The model under review builds one solid part; all positions refer to its coordinate system, in mm. Give positions to 0.01 mm unless a question says otherwise; leave off trailing zeros. Write each loop counter-clockwise with the first axis right and the second up, starting at its lowest first coordinate (ties: lowest second). Pieces come first, ordered by that corner, then holes. Notation, with made-up numbers: M -7,-10.75 L 33,-10.75 A20 cw 33,23.25 Z; hole C 81.5,63 d7. An arc over 180 degrees is marked long. Write item = value, one per line. Start each with the question number.
```python
from build123d import *

# Parameters (mm, degrees)
F0_R     = 2.5
F0_R_2   = 11.75
F1_DEPTH = 10


with BuildPart() as f1:
    # F0 (on Front) → F1 (new body)
    with BuildSketch(Plane.XZ):
        with BuildLine():
            Line((-30.310889, -27.5), (30.310889, -27.5))
            ThreePointArc((30.310889, -27.5), (38.971143, -22.5), (38.971143, -12.5))
            Line((38.971143, -12.5), (8.660254, 40))
            ThreePointArc((8.660254, 40), (0, 45), (-8.660254, 40))
            Line((-8.660254, 40), (-38.971143, -12.5))
            ThreePointArc((-38.971143, -12.5), (-38.971143, -22.5), (-30.310889, -27.5))
        make_face()
        with Locations((-30, -17.321524)):
            Circle(F0_R, mode=Mode.SUBTRACT)
        with Locations((30, -17.321524)):
            Circle(F0_R, mode=Mode.SUBTRACT)
        Circle(F0_R_2, mode=Mode.SUBTRACT)
        with Locations((0, 34.64)):
            Circle(F0_R, mode=Mode.SUBTRACT)
    extrude(amount=F1_DEPTH)


solid = f1.part
```
Item 1: Clearance check with flat-ended pins moving along their axes: P1, Ø1.5, axis at y = -1.5, z = -17, coming from the +X side; P2, Ø1.5, axis at y = -1, z = 0, coming from the -X side; P3, Ø1, axis at x = -10, y = -5.5, coming from the +Z side; P4, Ø3, axis at x = -3.5, y = -6, coming from the +Z side. State where each tip first meets the part, or that it passes through.
Item 2: The part is to be moulded in two halves that separate along Z. For faces 1 (the cylindrical face through (11.207, -4.93, 3.529)), 2 (the flat face through (0, -5, -27.5)), 3 (the flat face through (-23.6, -4.93, 14.12)), 4 (the flat face through (8, 0, 9)), say which applies: released by +Z, released by -Z, zero draft, split by the parting line, or undercut.
Item 3: We need section A-A, the plane x = 0. Write out the cut boundary in (y, z), and give its area (3 significant figures).
Item 4: We need section C-C, the plane x = -29. Write out the cut boundary in (y, z), and give its area (3 significant figures).
Item 5: We need section D-D, the plane z = 8. Write out the cut boundary in (x, y), and give its area (3 significant figures).
Item 6: We need section B-B, the plane z = -18.5. Write out the cut boundary in (x, y).
Item 7: To check wall thickness, follow probe 1 along Z at (x, y) = (1.5, -5); probe 2 along Z at (x, y) = (-30, -4); probe 3 along Z at (x, y) = (-28.5, -1.25). State the ranges of each line that lie inside material, in increasing order. Write a range as [from, to].
Worked out:
q1.P1 = 40.31
q1.P2 = -32.19
q1.P3 = 38.55
q1.P4 = 44.8
q2.face_1 = undercut
q2.face_2 = released by -Z
q2.face_3 = released by +Z
q2.face_4 = zero draft
q3.outline = M -10,-27.5 L 0,-27.5 L 0,-11.75 L -10,-11.75 Z; M -10,11.75 L 0,11.75 L 0,32.14 L -10,32.14 Z; M -10,37.14 L 0,37.14 L 0,45 L -10,45 Z
q3.area = 440 mm²
q4.outline = M -10,-27.5 L 0,-27.5 L 0,-19.61 L -10,-19.61 Z; M -10,-15.03 L 0,-15.03 L 0,4.77 L -10,4.77 Z
q4.area = 277 mm²
q5.outline = M -27.14,-10 L -8.61,-10 L -8.61,0 L -27.14,0 Z; M 8.61,-10 L 27.14,-10 L 27.14,0 L 8.61,0 Z
q5.area = 371 mm²
q6.outline = M -40.26,-10 L -32.2,-10 L -32.2,0 L -40.26,0 Z; M -27.8,-10 L 27.8,-10 L 27.8,0 L -27.8,0 Z; M 32.2,-10 L 40.26,-10 L 40.26,0 L 32.2,0 Z
q7.probe_1 = [-27.5, -11.65], [11.65, 32.64], [36.64, 44.89]
q7.probe_2 = [-27.5, -19.82], [-14.82, 3.04]
q7.probe_3 = [-27.5, -19.32], [-15.32, 5.64]
